Verification items for the finished model (mm, model axes). A direction names the side the tool comes from. Round coordinates to 2 decimals unless told otherwise and drop trailing zeros. Write each loop counter-clockwise with the first axis right and the second up, starting at its lowest first coordinate (ties: lowest second). Pieces come first, ordered by that corner, then holes. Notation, with made-up numbers: (41, -18.75) - (50, -18.75) arc R22 cw to (50, 13.25) - close; hole circle Ø10 at (23.5, -20). An arc over 180 degrees is marked (long way). Answer as a JSON object with one key per item and string values.
```python
from build123d import *

# Parameters (mm, degrees)
CUT_EXTRUDE_START        = -15
CUT_EXTRUDE_1_DEPTH      = 15
PATTERN_CIRCULAR_1_COUNT = 3


with BuildPart() as part:
    # Sketch 2 → Revolve 1 (revolve)
    with BuildSketch(Plane.XY, mode=Mode.PRIVATE) as revolve_1_sk:
        Polygon((3, 0), (48, 0), (48, 12), (46, 12), (40, 6), (10, 6), (10, 26), (5.5, 26), (5.5, 23), (3, 23), align=None)
    revolve(revolve_1_sk.sketch.rotate(Axis((0, -31.681818182, 0), (0, 1, 0)), 90), axis=Axis((0, -31.681818182, 0), (0, 1, 0)))

    # Sketch 4 → Cut-Extrude 1 (cut)
    with BuildSketch(Plane(origin=(0, 0, 0), x_dir=(-1, 0, 0), z_dir=(0, -1, 0)).offset(CUT_EXTRUDE_START)):
        with BuildLine():
            Line((-18.577383711, 20), (43.634848459, 20))
            ThreePointArc((43.634848459, 20), (43.159739663, 21.005639058), (42.661458015, 22))
            Line((42.661458015, 22), (-18.577383711, 22))
            ThreePointArc((-18.577383711, 22), (-31.5, 21), (-18.577383711, 20))
        make_face()
    cut_extrude_1 = extrude(amount=CUT_EXTRUDE_1_DEPTH, mode=Mode.SUBTRACT)

    # Pattern Circular 1: Cut-Extrude 1 ×3 about axis
    pattern_circular_1_axis = Axis((0, 0, 0), (0, 1, 0))
    for i in range(1, PATTERN_CIRCULAR_1_COUNT):
        add(cut_extrude_1.rotate(pattern_circular_1_axis, i * 360 / PATTERN_CIRCULAR_1_COUNT), mode=Mode.SUBTRACT)


solid = part.part
```
Q1. Section check B-B, the plane z = 0. Record the cut outline in (x, y), then the cut area to 3 significant figures.
Geometry check:
{"outline": "(-48, 0) - (-25.4, 0) - (-25.4, 6) - (-40, 6) - (-46, 12) - (-48, 12) - close; (-23.09, 0) - (-3, 0) - (-3, 23) - (-5.5, 23) - (-5.5, 26) - (-10, 26) - (-10, 6) - (-23.09, 6) - close; (3, 0) - (23.09, 0) - (23.09, 6) - (10, 6) - (10, 26) - (5.5, 26) - (5.5, 23) - (3, 23) - close; (25.4, 0) - (48, 0) - (48, 12) - (46, 12) - (40, 6) - (25.4, 6) - close", "area": "837 mm2"}
Q2. Gauge pin test, flat ends, axial feed: P1, Ø13, axis at x = -27, y = 5.5, coming from the +Z side; P2, Ø5, axis at x = -29, y = 11, coming from the -Z side; P3, Ø22.5, axis at x = 14.5, z = 29.5, coming from the +Y side. Record the tip position at first contact, or that the pin passes through.
Geometry check:
{"P1": "stops at z = 43.4", "P2": "stops at z = -40.02", "P3": "stops at y = 10.12"}
Q3. Material ranges on line 1 along X through (y, z) = (14.75, 0); line 2 along Z through (x, y) = (25, 2.75); line 3 along X through (y, z) = (4, 14.5), recorded low to high. Write a range as [from, to].
Geometry check:
{"line 1": "x = [-10, -3], [3, 10]", "line 2": "z = [-40.98, -27.5], [-14.5, -3.3], [0.7, 40.98]", "line 3": "x = [-45.76, -17.03], [-14.72, 14.72], [17.03, 45.76]"}
Q4. Set-up check for faces 5 (the cylindrical face through (42.854, 6.084, 21.622)), 6 (the conical face through (0.1, 6.3, -40.3)), 7 (the flat face through (-12.817, 3.417, 21.8)), 8 (the flat face through (-38, 12, 27)), 9 (the flat face through (10, 0, -1)): record each of +Z, -Z, +X, -X, +Y, -Y from which the full face is reachable in a straight line by a thin tool's end or side.
Geometry check:
{"face 5": "+X, +Y, -Y", "face 6": "+Y", "face 7": "+Y, -Y", "face 8": "+Z, -X, +Y", "face 9": "+Z, -Z, +X, -X, -Y"}
Q5. Release check for a two-part mould opening along Z. For faces 1 (the flat face through (-12, 3, -20)), 2 (the flat face through (-2, 12, -46.5)), 3 (the cylindrical face through (-40.152, 6.084, 26.302)), 4 (the cylindrical face through (-2.702, 6.084, -47.924)) record: released by +Z, released by -Z, zero draft, split by the parting line, or undercut.
Geometry check:
{"face 1": "undercut", "face 2": "zero draft", "face 3": "split by the parting line", "face 4": "released by -Z"}
Q6. Section check C-C, the plane z = 21. State how many separate pieces and enclosed holes the cut face has, then the cut area to 3 significant figures.
Geometry check:
{"separate pieces": "3", "enclosed holes": "0", "area": "558 mm2"}
Q7. Section check A-A, the plane y = 2.25. Record the cut outline in (x, z).
Geometry check:
{"outline": "(-43.63, -20) - (18.58, -20) arc R6.5 cw (long way) to (18.58, -22) - (-42.66, -22) arc R48 ccw to (39.14, -27.79) - (8.03, 26.09) arc R6.5 cw (long way) to (9.76, 27.09) - (40.38, -25.95) arc R48 ccw to (4.5, 47.79) - (-26.61, -6.09) arc R6.5 cw (long way) to (-28.34, -5.09) - (2.28, 47.95) arc R48 ccw to start; hole circle Ø6 at (0, 0)"}
